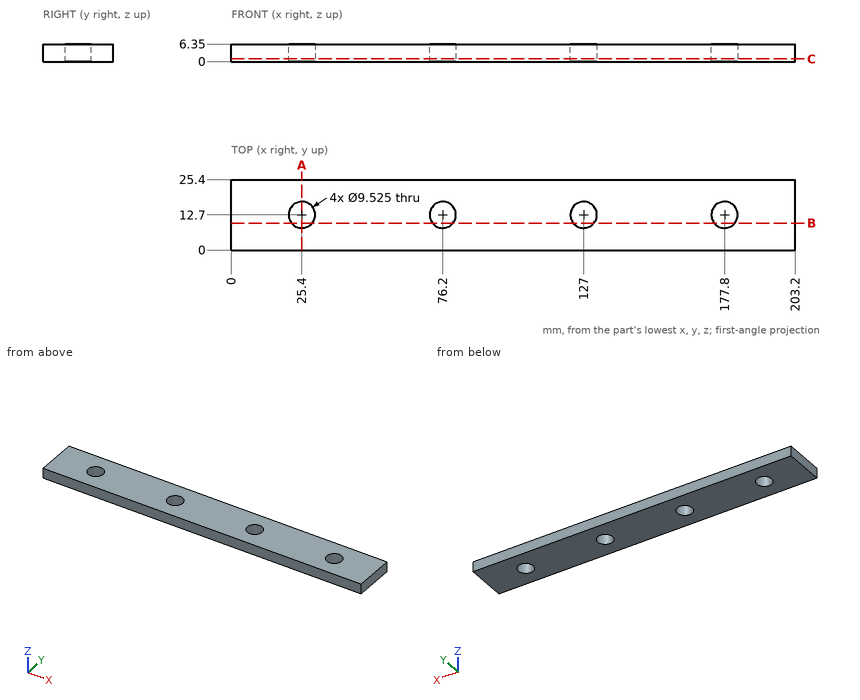
Input: dimensioned drawing with shaded views. Units: mm. Origin: part minimum x, y, z. Give positions to 0.01 mm unless a question says otherwise; leave off trailing zeros. Loops run counter-clockwise (first coordinate to the right, second up) from the corner with the lowest first, then second, coordinate; pieces in that order, holes last. Notation, with made-up numbers: M 34.5,72 L 65.5,72 A32 cw 65.5,102 Z; hole C 33,-33.5 d11. An arc over 180 degrees is marked long. Put each result on its own line as item: value. Start each with the question number.
1) Cut plane A-A (x = 25.4). Output: boundary loops of the cut face in (y, z), then the cut area to 3 significant figures.
2) Ray query, line 1 along Y through (x, z) = (177.8, 5); line 2 along X through (y, z) = (9.5, 4.5); line 3 along X through (y, z) = (8.5, 5.75). Return the intervals inside material, ascending.
3) Cut plane C-C (z = 1). Output: boundary loops of the cut face in (x, y) (1 decimal).
4) Contact query for a flat-ended pin moving along its axis: pin 1 (5.5 mm diameter, centred on x = 127, y = 12.7, fed in from -Z). Output: stop coordinate, or through.
5) Cut plane B-B (y = 9.75). Output: boundary loops of the cut face in (x, z).
Verdict:
1. outline: M 0,0 L 7.94,0 L 7.94,6.35 L 0,6.35 Z; M 17.46,0 L 25.4,0 L 25.4,6.35 L 17.46,6.35 Z
1. area: 101 mm2
2. line 1: 0 to 7.94, 17.46 to 25.4
2. line 2: 0 to 21.87, 28.93 to 72.67, 79.73 to 123.47, 130.53 to 174.27, 181.33 to 203.2
2. line 3: 0 to 23.15, 27.65 to 73.95, 78.45 to 124.75, 129.25 to 175.55, 180.05 to 203.2
3. outline: M 0,0 L 203.2,0 L 203.2,25.4 L 0,25.4 Z; hole C 25.4,12.7 d9.5; hole C 76.2,12.7 d9.5; hole C 127,12.7 d9.5; hole C 177.8,12.7 d9.5
4. pin 1: through
5. outline: M 0,0 L 21.66,0 L 21.66,6.35 L 0,6.35 Z; M 29.14,0 L 72.46,0 L 72.46,6.35 L 29.14,6.35 Z; M 79.94,0 L 123.26,0 L 123.26,6.35 L 79.94,6.35 Z; M 130.74,0 L 174.06,0 L 174.06,6.35 L 130.74,6.35 Z; M 181.54,0 L 203.2,0 L 203.2,6.35 L 181.54,6.35 Z
